Here's the drawing with two shaded views (mm, measured from the low corner). I have some questions. A direction names the side the tool comes from. Round coordinates to 2 decimals unless told otherwise and drop trailing zeros. Loops run counter-clockwise (first coordinate to the right, second up) from the corner with the lowest first, then second, coordinate; pieces in that order, holes last. Notation, with made-up numbers: (-7, 62.5) -> (3, 62.5) arc R33 ccw to (3, 97.5) -> close; hole circle Ø6 at (25, -3.75). An arc over 180 degrees is marked (long way). One line per item, written item: value. Start each with the question number.
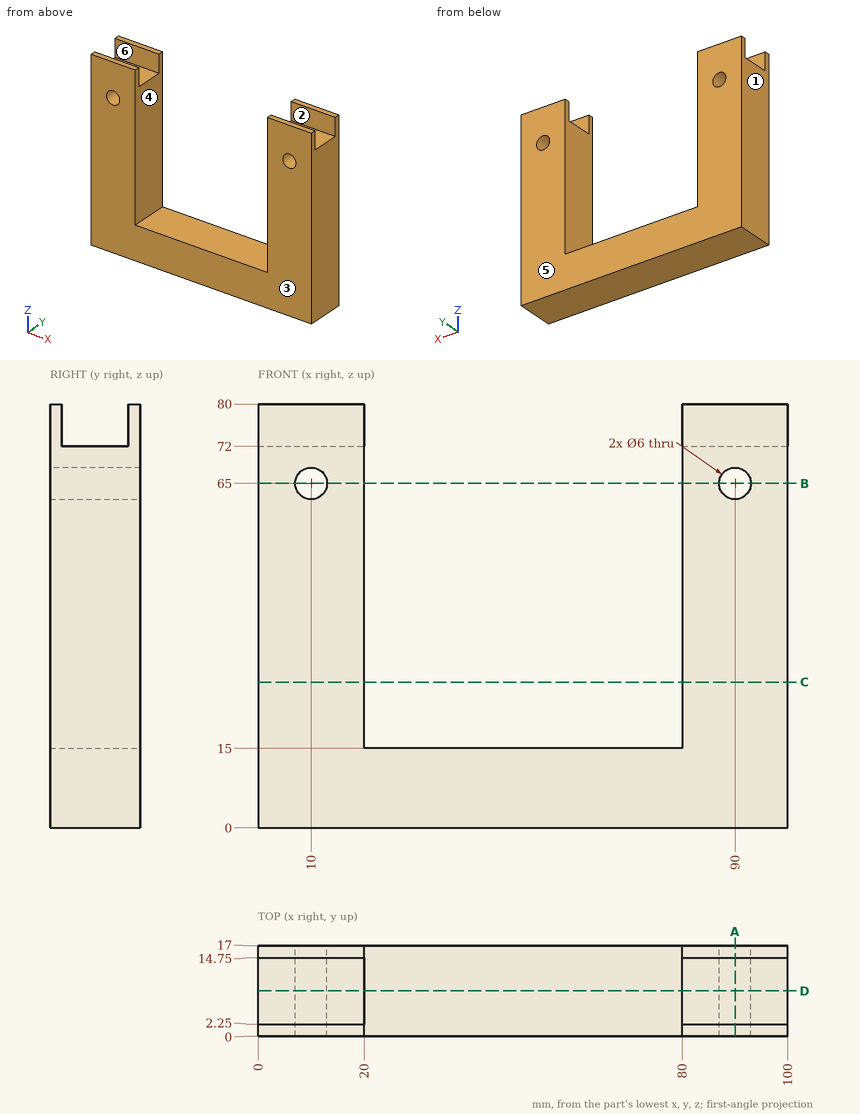
Q1. I want a section at B-B on z = 65. Please give me the cut outline in (x, y).
Q2. I want a section at D-D on y = 8.5. Please give me the cut outline in (x, z).
Q3. Will this pin go through, and if not, where does the flat tip stop? P1, Ø10, axis at x = 87, y = 9, coming from the +Z side.
Q4. If I drill on line 1 along X through (y, z) = (11.5, 65); line 2 along Z through (x, y) = (90, 10.25); line 3 along X through (y, z) = (5, 61), over which ranges is the centre line in solid material (lowest first)?
Q5. I want a section at C-C on z = 27.5. Please give me the cut outline in (x, y), plus the area to 3 significant figures.
Q6. I want a section at A-A on x = 90. Please give me the cut outline in (y, z).
Q7. If we mould it in two halves opening along Y, with no side actions, what happens to the marked faces 1, 2 and 3? For each: released by +Y, released by -Y, zero draft, split by the parting line, or undercut.
Q8. Which directions (+Z, -Z, +X, -X, +Y, -Y) give clear straight access to the entire face, cutting with the end or side of a thin tool? Please do the marked faces 4, 5 and 6.
Answers below:
1. outline: (0, 0) -> (7, 0) -> (7, 17) -> (0, 17) -> close; (13, 0) -> (20, 0) -> (20, 17) -> (13, 17) -> close; (80, 0) -> (87, 0) -> (87, 17) -> (80, 17) -> close; (93, 0) -> (100, 0) -> (100, 17) -> (93, 17) -> close
2. outline: (0, 0) -> (100, 0) -> (100, 72) -> (80, 72) -> (80, 15) -> (20, 15) -> (20, 72) -> (0, 72) -> close; hole circle Ø6 at (10, 65); hole circle Ø6 at (90, 65)
3. P1: stops at z = 72
4. line 1: x = 0 to 7, 13 to 20, 80 to 87, 93 to 100
4. line 2: z = 0 to 62, 68 to 72
4. line 3: x = 0 to 20, 80 to 100
5. outline: (0, 0) -> (20, 0) -> (20, 17) -> (0, 17) -> close; (80, 0) -> (100, 0) -> (100, 17) -> (80, 17) -> close
5. area: 680 mm^2
6. outline: (0, 0) -> (17, 0) -> (17, 62) -> (0, 62) -> close; (0, 68) -> (17, 68) -> (17, 80) -> (14.75, 80) -> (14.75, 72) -> (2.25, 72) -> (2.25, 80) -> (0, 80) -> close
7. face 1: zero draft
7. face 2: undercut
7. face 3: released by -Y
8. face 4: +Z, +Y, -Y
8. face 5: +Z, -Z, +X, -X, +Y
8. face 6: +Z, +X, -X
